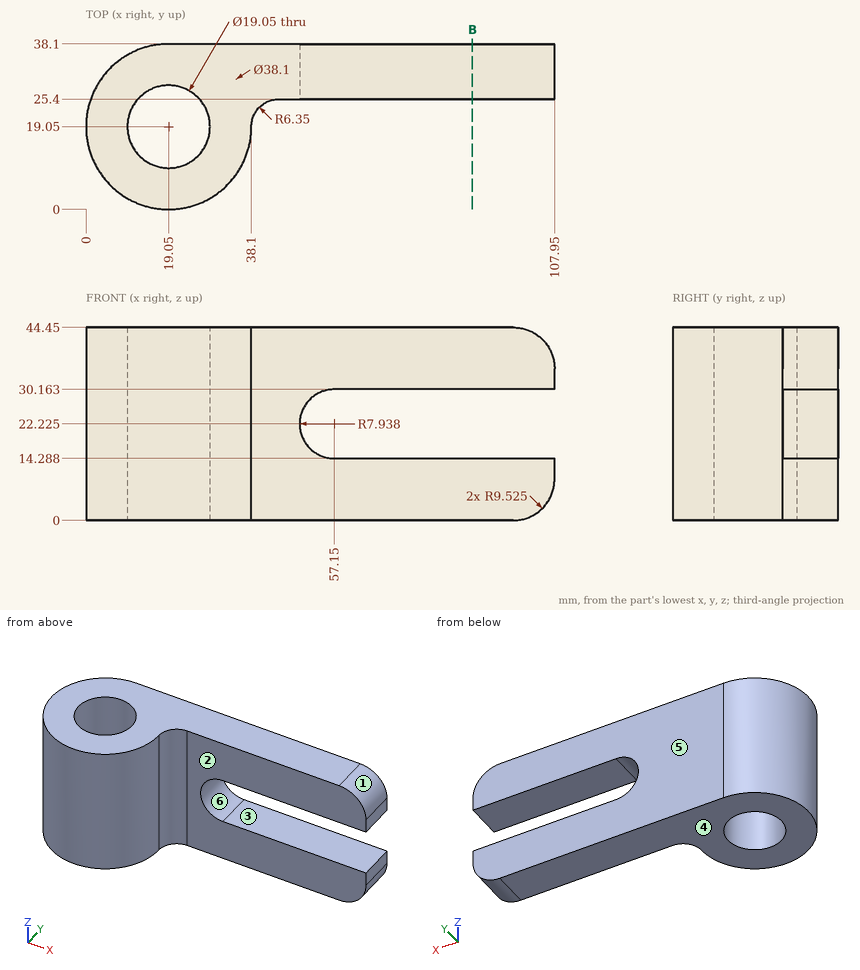
Geometry check sheet. Reference: drawing and pictorial views, mm from the part's lowest x, y, z. A direction names the side the tool comes from. Coordinates: 2 decimals unless noted, no trailing zeros. Order: outer loops, then holes, each group sorted by start corner. A loop starts at its lowest first (then second) coordinate and runs counter-clockwise, first axis right, second up.
1. Sectioned sample at B-B, the plane x = 89. Record the cut outline in (y, z), and give its area (3 significant figures).
Results found:
outline: (25.4, 0) - (38.1, 0) - (38.1, 14.29) - (25.4, 14.29) - close; (25.4, 30.16) - (38.1, 30.16) - (38.1, 44.45) - (25.4, 44.45) - close
area: 363 mm2
2. Go/stop test with flat-tipped pins: pin 1 Ø4 at (y, z) = (24.5, 35) entering from -X (1 decimal); pin 2 Ø4 at (y, z) = (9, 7) entering from +X (1 decimal); pin 3 Ø4 at (x, z) = (92, 30.5) entering from -Y. Record where each tip stops, or that it passes through.
Results found:
pin 1: stops at x = 0.3
pin 2: stops at x = 36.3
pin 3: stops at y = 25.4
3. Set-up check for the marked faces 1, 2 and 3: record each of +Z, -Z, +X, -X, +Y, -Y from which the full face is reachable in a straight line by a thin tool's end or side.
Results found:
face 1: +Z, +X, +Y, -Y
face 2: +Z, -Z, +X, -Y
face 3: +X, +Y, -Y
4. Scan lines: line 1 (Y direction, x = 19, z = 29) (1 decimal); line 2 (Z direction, x = 91, y = 36). Record each from-to range of solid material in increasing order.
Results found:
line 1: y = 0 to 9.5, 28.6 to 38.1
line 2: z = 0 to 14.29, 30.16 to 44.45
5. Release check for a two-part mould opening along Z. For the marked faces 4, 5 and 6 record: +Z half, -Z half, draft (parallel to the pull), parting line (faces both ways), or undercut.
Results found:
face 4: -Z half
face 5: draft
face 6: undercut
